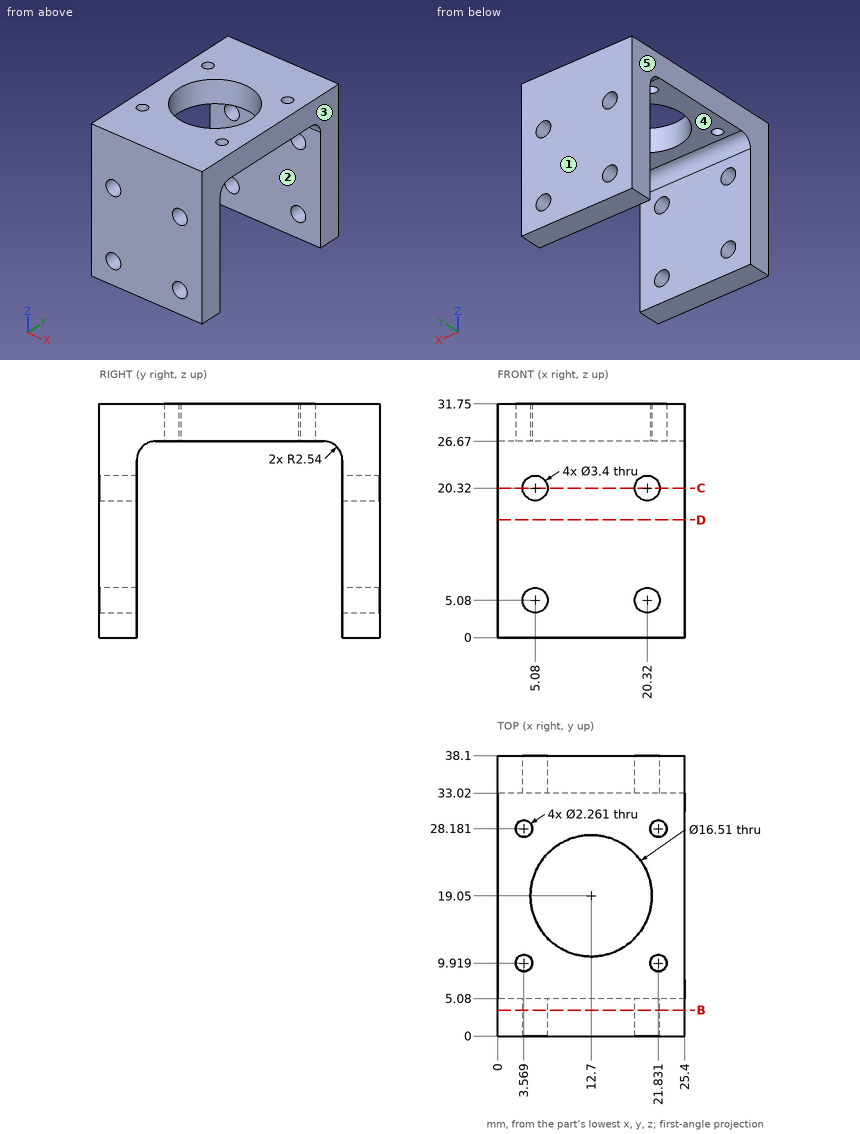
Geometry check sheet. Reference: drawing and pictorial views, mm from the part's lowest x, y, z. A direction names the side the tool comes from. Coordinates: 2 decimals unless noted, no trailing zeros. Order: outer loops, then holes, each group sorted by start corner. A loop starts at its lowest first (then second) coordinate and runs counter-clockwise, first axis right, second up. Notation, with made-up numbers: (34, -15) - (71, -15) arc R5 cw to (71, -7) - close; hole circle Ø3 at (-9, 44.5). An arc over 180 degrees is marked (long way). One line per item, written item: value.
(1) Access from +Z, -Z, +X, -X, +Y, -Y to the whole of each face (thin tool, end or side, straight path). Record for the marked faces 4 and 5.
Data:
face 4: -Z, +X, -X
face 5: +Z, -Z, -X, +Y, -Y
(2) Sectioned sample at D-D (z = 16). Enter the section's corners in (x, y).
Data:
outline: (0, 0) - (25.4, 0) - (25.4, 5.08) - (0, 5.08) - close; (0, 33.02) - (25.4, 33.02) - (25.4, 38.1) - (0, 38.1) - close
(3) Sectioned sample at C-C (z = 20.32). Enter the section's corners in (x, y), and give its area (3 significant figures).
Data:
outline: (0, 0) - (3.38, 0) - (3.38, 5.08) - (0, 5.08) - close; (0, 33.02) - (3.38, 33.02) - (3.38, 38.1) - (0, 38.1) - close; (6.78, 0) - (18.62, 0) - (18.62, 5.08) - (6.78, 5.08) - close; (6.78, 33.02) - (18.62, 33.02) - (18.62, 38.1) - (6.78, 38.1) - close; (22.02, 0) - (25.4, 0) - (25.4, 5.08) - (22.02, 5.08) - close; (22.02, 33.02) - (25.4, 33.02) - (25.4, 38.1) - (22.02, 38.1) - close
area: 189 mm^2
(4) Depth check by flat-ended pin: pin 1 Ø8 at (x, y) = (22, 18) entering from -Z. Enter the tip coordinate at first touch or a pass-through.
Data:
pin 1: stops at z = 26.67
(5) Sectioned sample at B-B (y = 3.5). Enter the section's corners in (x, z), and give its area (3 significant figures).
Data:
outline: (0, 0) - (25.4, 0) - (25.4, 31.75) - (0, 31.75) - close; hole circle Ø3.4 at (5.08, 5.08); hole circle Ø3.4 at (5.08, 20.32); hole circle Ø3.4 at (20.32, 5.08); hole circle Ø3.4 at (20.32, 20.32)
area: 770 mm^2
(6) Thickness scan on probe 1 along X at (y, z) = (2.3, 5.08); probe 2 along Y at (x, z) = (23.75, 13.5); probe 3 along Z at (x, y) = (4.5, 5). Record the ranges inside material, lowest first. Write a range as from..to.
Data:
probe 1: x = 0..3.38, 6.78..18.62, 22.02..25.4
probe 2: y = 0..5.08, 33.02..38.1
probe 3: z = 0..3.48, 6.68..18.72, 21.92..31.75
(7) Release check for a two-part mould opening along Y. For the marked faces 1, 2 and 3 record: +Y half, -Y half, draft (parallel to the pull), parting line (faces both ways), or undercut.
Data:
face 1: +Y half
face 2: undercut
face 3: draft
